Source: CAD feature listing. Evaluate the final solid. Frame: model axes, mm. Round coordinates to 2 decimals unless told otherwise and drop trailing zeros. Loops run counter-clockwise (first coordinate to the right, second up) from the corner with the lowest first, then second, coordinate; pieces in that order, holes last. Notation, with made-up numbers: (53, -13) - (72, -13) arc R30 cw to (72, 24) - close; hole circle Ø4 at (20.5, 2.25). An arc over 180 degrees is marked (long way). One line per question, with ' | ' between items. Start each with the question number.
1. Cut plane C-C (x = -13). Return loops of the section in (y, z).
2. Cut plane B-B (z = 0). Return loops of the section in (x, y), then the cut area to 3 significant figures.
3. Cut plane A-A (y = -3). Return loops of the section in (x, z).
4. Cut plane D-D (y = -6.5). Return loops of the section in (x, z), then the cut area to 3 significant figures.
5. Ray query, line 1 (X direction, y = -0.25, z = 0.75); line 2 (Y direction, x = -17.5, z = -1.75); line 3 (Y direction, x = 20, z = 4.75). Return the intervals inside material, ascending.
6. Pin query (flat end, axial travel): pin 1 (4 mm diameter, centred on x = -11, z = 0.5, fed in from -Y); pin 2 (5 mm diameter, centred on y = 2.5, z = -3, fed in from -X); pin 3 (2 mm diameter, centred on y = 2.5, z = -3.5, fed in from +X). Return the tip coordinate at first contact, or that it passes through.
```python
from build123d import *

# Parameters (mm, degrees)
SKETCH_1_W        = 47
SKETCH_1_H        = 10
EXTRUDE_1_DEPTH   = 5
CHAMFER_1_SIZE    = 1
SWEEP_1_PROFILE_R = 0.5
SWEEP_2_PROFILE_R = 0.5


with BuildPart() as part:
    # 草图1 → 凸台-拉伸1 (new, symmetric)
    with BuildSketch(Plane(origin=(0, 0, 0), x_dir=(1, 0, 0), z_dir=(0, 1, 0))):
        Rectangle(SKETCH_1_W, SKETCH_1_H)
    extrude(amount=EXTRUDE_1_DEPTH, both=True)

    # 倒角1
    chamfer_1_edges = [part.edges().sort_by_distance(p)[0] for p in [
        (-23.5, 5, 0),
        (0, 5, 5),
        (23.5, 5, 0),
        (0, -5, 5),
        (-23.5, -5, 0),
        (0, -5, -5),
        (23.5, -5, 0),
        (0, 5, -5),
    ]]
    chamfer(chamfer_1_edges, length=CHAMFER_1_SIZE)

    # 扫描1: sweep along a path in 草图2
    with BuildLine(Plane.XY) as sweep_1_path:
        Line((23.5, 0), (24.5, 0))
        ThreePointArc((24.5, 0), (25.207106781, -0.292893219), (25.5, -1))
        Line((25.5, -1), (25.5, -8))
    # 扫描1 profile (on start of the path) → 扫描1 (sweep)
    with BuildSketch(Plane.YZ.offset(23.5)):
        Circle(SWEEP_1_PROFILE_R)
    sweep(path=sweep_1_path.line)

    # 扫描2: sweep along a path in 草图9
    with BuildLine(Plane.XY) as sweep_2_path:
        Line((-23.5, 0), (-24.5, 0))
        ThreePointArc((-24.5, 0), (-25.207106781, -0.292893219), (-25.5, -1))
        Line((-25.5, -1), (-25.5, -8))
    # 扫描2 profile (on start of the path) → 扫描2 (sweep)
    with BuildSketch(Plane(origin=(-23.5, 0, 0), x_dir=(0, -1, 0), z_dir=(-1, 0, 0))):
        Circle(SWEEP_2_PROFILE_R)
    sweep(path=sweep_2_path.line)


solid = part.part
```
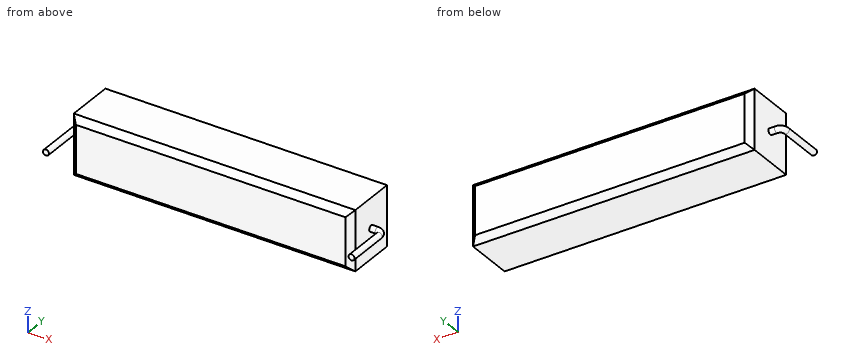
Answers follow:
1) outline: (-5, -4) - (-4, -5) - (4, -5) - (5, -4) - (5, 4) - (4, 5) - (-4, 5) - (-5, 4) - close
2) outline: (-26, -8) - (-25, -8) - (-25, -1) arc R0.5 cw to (-24.5, -0.5) - (-23.5, -0.5) - (-23.5, -4) - (-22.5, -5) - (22.5, -5) - (23.5, -4) - (23.5, -0.5) - (24.5, -0.5) arc R0.5 cw to (25, -1) - (25, -8) - (26, -8) - (26, -1) arc R1.5 ccw to (24.5, 0.5) - (23.5, 0.5) - (23.5, 4) - (22.5, 5) - (-22.5, 5) - (-23.5, 4) - (-23.5, 0.5) - (-24.5, 0.5) arc R1.5 ccw to (-26, -1) - close | area: 487 mm2
3) outline: circle Ø1 at (-25.5, 0); (-23.5, -5) - (23.5, -5) - (23.5, 5) - (-23.5, 5) - close; circle Ø1 at (25.5, 0)
4) outline: circle Ø1 at (-25.5, 0); circle Ø1 at (25.5, 0) | area: 1.57 mm2
5) line 1: x = -23.5 to 23.5 | line 2: y = -5 to 5 | line 3: y = -4.25 to 4.25
6) pin 1: stops at y = -5 | pin 2: stops at x = -23.5 | pin 3: stops at x = 23.5
